```python
from build123d import *

# Parameters (mm, degrees)
F0_W     = 31.75
F0_H     = 15.75
F0_W_2   = 30.05
F0_H_2   = 14.05
F1_DEPTH = 1
F2_DEPTH = 8.5


with BuildPart() as f1:
    # F0 (on Front) → F1 (new body)
    with BuildSketch(Plane.XZ):
        Rectangle(F0_W, F0_H)
        Rectangle(F0_W_2, F0_H_2, mode=Mode.SUBTRACT)
        Rectangle(F0_W_2, F0_H_2)
    extrude(amount=F1_DEPTH)

    # F0 (on Front) → F2 (join)
    with BuildSketch(Plane.XZ):
        Rectangle(F0_W, F0_H)
        Rectangle(F0_W_2, F0_H_2, mode=Mode.SUBTRACT)
    extrude(amount=F2_DEPTH)


solid = f1.part
```
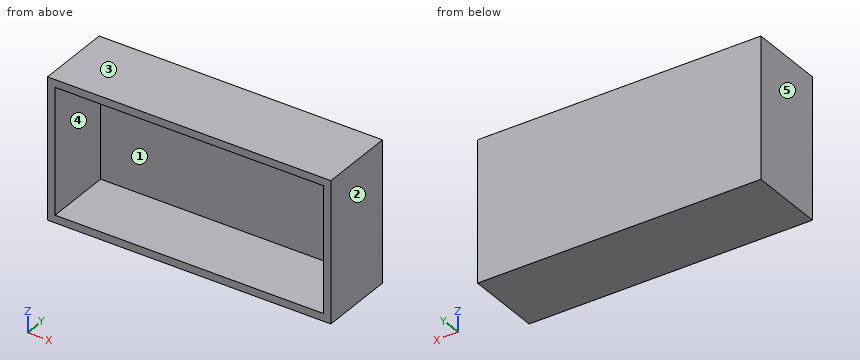
The model under review builds one solid part; all positions refer to its coordinate system, in mm. Face numbers are marked on the shaded views. A direction names the side the tool comes from. Round coordinates to 2 decimals unless told otherwise and drop trailing zeros. Loops run counter-clockwise (first coordinate to the right, second up) from the corner with the lowest first, then second, coordinate; pieces in that order, holes last. Notation, with made-up numbers: M -31,-37 L -4,-37 A25 ccw -4,-9 Z; hole C 38,-17 d5. An arc over 180 degrees is marked long. Put each result on its own line as item: value.
Q1. Consider section C-C, the plane x = -9. Give the boundary of the cut face in (y, z) (3 decimals), then the cut area to 3 significant figures.
Result set:
outline: M -8.5,-7.875 L 0,-7.875 L 0,7.875 L -8.5,7.875 L -8.5,7.025 L -1,7.025 L -1,-7.025 L -8.5,-7.025 Z
area: 28.5 mm²
Q2. Consider section A-A, the plane y = -3. Give the boundary of the cut face in (x, z) (3 decimals).
Result set:
outline: M -15.875,-7.875 L 15.875,-7.875 L 15.875,7.875 L -15.875,7.875 Z; hole M -15.025,-7.025 L 15.025,-7.025 L 15.025,7.025 L -15.025,7.025 Z
Q3. Mouldability with a two-part tool opening along X and no side actions: class the marked faces 1, 2 and 3 as released by +X, released by -X, zero draft, split by the parting line, or undercut.
Result set:
face 1: undercut
face 2: released by +X
face 3: zero draft
Q4. Consider section B-B, the plane z = -0.25. Give the boundary of the cut face in (x, y) (3 decimals).
Result set:
outline: M -15.875,-8.5 L -15.025,-8.5 L -15.025,-1 L 15.025,-1 L 15.025,-8.5 L 15.875,-8.5 L 15.875,0 L -15.875,0 Z
Q5. Machinability: for the marked faces 4 and 5, which of the approach directions +Z, -Z, +X, -X, +Y, -Y give a long, thin tool a straight path to every point of the face, cutting with its end or side? Answer none if there is none.
Result set:
face 4: -Y
face 5: +Z, -Z, -X, +Y, -Y
Q6. To check wall thickness, follow L1, parallel to Z at x = 6.5, y = -2.5 (3 decimals); L2, parallel to X at y = -6.25, z = 3 (3 decimals); L3, parallel to Y at x = -8, z = 0. State the ranges of each line that lie inside material, in increasing order.
Result set:
L1: z = -7.875 to -7.025, 7.025 to 7.875
L2: x = -15.875 to -15.025, 15.025 to 15.875
L3: y = -1 to 0
Q7. For pin 1 (2 mm diameter, centred on x = 8, z = -4.5, fed in from -Y), flat-tipped, find the tip position at first contact; note if it passes through.
Result set:
pin 1: stops at y = -1
